The model under review builds one solid part; all positions refer to its coordinate system, in mm. A direction names the side the tool comes from. Coordinates: 2 decimals unless noted, no trailing zeros. Write each loop counter-clockwise with the first axis right and the second up, starting at its lowest first coordinate (ties: lowest second). Pieces come first, ordered by that corner, then holes.
1) Add section C-C, the plane y = -0.9. State the section outline as (x, z) points.
2) Add section D-D, the plane z = -9.25. State the section outline as (x, y) points, then the cut area to 3 significant figures.
3) For line 1 (X direction, y = 0.5, z = 3.5); line 2 (X direction, y = -1.7, z = 10); line 3 (Z direction, x = -26, y = -1.65), list the stretches that pass through material, from the lowest coordinate up.
4) For P1, Ø1.6, axis at x = 16, y = -1.5, coming from the +Z side; P2, Ø0.6, axis at y = -1, z = 3, coming from the -X side; P3, Ø5, axis at x = 13.5, z = -3, coming from the -Y side; P4, Ø1.5, axis at y = -0.5, z = 11, coming from the -X side, all flat-tipped, find the tip position at first contact; note any pin that passes through.
5) Add section A-A, the plane x = -30. State the section outline as (y, z) points.
6) Add section B-B, the plane z = 3.5. State the section outline as (x, y) points, then the cut area to 3 significant figures.
7) Machinability: for faces 4 (the flat face through (-1, 2, 0)), 5 (the flat face through (41, -1, 0)), 6 (the flat face through (-1, -1, 12.5)), 7 (the flat face through (-43, -1, 0)), which of the approach directions +Z, -Z, +X, -X, +Y, -Y give a long, thin tool a straight path to every point of the face, cutting with its end or side? Answer none if there is none.
8) Mouldability with a two-part tool opening along X and no side actions: class faces 1 (the flat face through (-1, -1, -12.5)), 2 (the flat face through (-1, -1, 10.5)), 3 (the flat face through (43, -1, 0)) as released by +X, released by -X, zero draft, split by the parting line, or undercut.
from build123d import *

# Parameters (mm, degrees)
SKETCH1_W           = 90
SKETCH1_H           = 29
BOSS_EXTRUDE1_DEPTH = 2
CHAMFER1_SIZE       = 1
SKETCH2_R           = 6.75
CUT_EXTRUDE1_DEPTH  = 48.32071428
SKETCH3_W           = 86
SKETCH3_H           = 25
SKETCH3_W_2         = 82
SKETCH3_H_2         = 21
BOSS_EXTRUDE2_DEPTH = 2


with BuildPart() as part:
    # Sketch1 → Boss-Extrude1 (new body)
    with BuildSketch(Plane(origin=(0, 0, 0), x_dir=(1, 0, 0), z_dir=(0, 1, 0))):
        Rectangle(SKETCH1_W, SKETCH1_H)
    extrude(amount=BOSS_EXTRUDE1_DEPTH)

    # Chamfer1
    chamfer1_edges = [part.edges().sort_by_distance(p)[0] for p in [
        (-45, 2, 0),
        (0, 2, 14.5),
        (45, 2, 0),
        (45, 1, 14.5),
        (-45, 1, 14.5),
        (-45, 1, -14.5),
        (45, 1, -14.5),
        (0, 2, -14.5),
    ]]
    chamfer(chamfer1_edges, length=CHAMFER1_SIZE)

    # Sketch2 → Cut-Extrude1 (cut, through all)
    with BuildSketch(Plane(origin=(0, 2, 0), x_dir=(1, 0, 0), z_dir=(0, 1, 0))):
        with Locations(Location((-30, -3.5, 0), (0, 0, 270))):
            Circle(SKETCH2_R)
        with Locations(Location((30, -3.5, 0), (0, 0, 270))):
            Circle(SKETCH2_R)
    extrude(amount=-CUT_EXTRUDE1_DEPTH, mode=Mode.SUBTRACT)

    # Sketch3 → Boss-Extrude2 (add)
    with BuildSketch(Plane.XZ):
        Rectangle(SKETCH3_W, SKETCH3_H)
        Rectangle(SKETCH3_W_2, SKETCH3_H_2, mode=Mode.SUBTRACT)
    extrude(amount=BOSS_EXTRUDE2_DEPTH)


solid = part.part
Geometry results:
1. outline: (-43, -12.5) - (43, -12.5) - (43, 12.5) - (-43, 12.5) - close; hole (-41, -10.5) - (41, -10.5) - (41, 10.5) - (-41, 10.5) - close
2. outline: (-45, 0) - (-43, 0) - (-43, -2) - (-41, -2) - (-41, 0) - (41, 0) - (41, -2) - (43, -2) - (43, 0) - (45, 0) - (45, 1) - (44, 2) - (-44, 2) - (-45, 1) - close
2. area: 187 mm2
3. line 1: x = -45 to -36.75, -23.25 to 23.25, 36.75 to 45
3. line 2: x = -43 to -41, 41 to 43
3. line 3: z = -12.5 to -10.5, 10.5 to 12.5
4. P1: stops at z = 12.5
4. P2: stops at x = -43
4. P3: stops at y = 0
4. P4: stops at x = -45
5. outline: (-2, -12.5) - (0, -12.5) - (0, -14.5) - (1, -14.5) - (2, -13.5) - (2, -3.25) - (0, -3.25) - (0, -10.5) - (-2, -10.5) - close; (-2, 10.5) - (0, 10.5) - (0, 10.25) - (2, 10.25) - (2, 13.5) - (1, 14.5) - (0, 14.5) - (0, 12.5) - (-2, 12.5) - close
6. outline: (-45, 0) - (-43, 0) - (-43, -2) - (-41, -2) - (-41, 0) - (-36.75, 0) - (-36.75, 2) - (-44, 2) - (-45, 1) - close; (-23.25, 0) - (23.25, 0) - (23.25, 2) - (-23.25, 2) - close; (36.75, 0) - (41, 0) - (41, -2) - (43, -2) - (43, 0) - (45, 0) - (45, 1) - (44, 2) - (36.75, 2) - close
6. area: 133 mm2
7. face 4: +Z, -Z, +X, -X, +Y
7. face 5: -Y
7. face 6: +Z, +X, -X, -Y
7. face 7: +Z, -Z, -X, -Y
8. face 1: zero draft
8. face 2: undercut
8. face 3: released by +X
